Design review of the part built by this model. Coordinates are the model's own, in mm. A direction names the side the tool comes from. Round coordinates to 2 decimals unless told otherwise and drop trailing zeros. Write each loop counter-clockwise with the first axis right and the second up, starting at its lowest first coordinate (ties: lowest second). Pieces come first, ordered by that corner, then holes. Notation, with made-up numbers: (32.25, 3) -> (41.25, 3) arc R24 ccw to (41.25, 18) -> close; hole circle Ø6 at (66, -22). An arc over 180 degrees is marked (long way). One line per question, with ' | ' between items. Start each with the question number.
1) For probe 1 along Y at (x, z) = (3, -3.5); probe 2 along Y at (x, z) = (4, -10); probe 3 along Z at (x, y) = (-0.5, -2.25), list the stretches that pass through material, from the lowest coordinate up.
2) Insertion check: pin 1 Ø2.5 at (y, z) = (5.5, 12) entering from -X; pin 2 Ø4 at (y, z) = (2.5, -4.5) entering from +X; pin 3 Ø2 at (x, z) = (4, -3.5) entering from +Y; pin 4 Ø5 at (x, y) = (5, 6.5) entering from -Z. Each pin has a flat end and moves straight along its axis. Give the tip position at first contact, or say it passes through.
3) Consider section D-D (z = -14.5). Give the boundary of the cut face in (x, y).
4) Mouldability with a two-part tool opening along X and no side actions: class faces 4 (the flat face through (12, 2, 5)), 5 (the flat face through (-15, 6, 0)), 6 (the flat face through (-15, -2, 0)) as +X half, -X half, draft (parallel to the pull), parting line (faces both ways), or undercut.
5) Consider section C-C (y = 2.25). Give the boundary of the cut face in (x, z), then the cut area to 4 significant figures.
6) Consider section B-B (x = -10.5). Give the boundary of the cut face in (y, z), then the cut area to 3 significant figures.
7) Consider section A-A (y = 5.5). Give the boundary of the cut face in (x, z), then the cut area to 3 significant figures.
8) For faces 1 (the flat face through (0, 6, -15)), 2 (the flat face through (0, -1, 2)), 3 (the flat face through (-12, 2, 5)), list the 3-axis set-ups (+Z, -Z, +X, -X, +Y, -Y) from which the entire face can be reached by the end or side of a thin tool; tool diameter is ignored.
```python
from build123d import *

# Parameters (mm, degrees)
SKETCH1_W                = 10
SKETCH1_H                = 15
BOSS_EXTRUDE1_DEPTH      = 4
BOSS_EXTRUDE6_DEPTH      = 8
BOSS_EXTRUDE5_DEPTH      = 15
BOSS_EXTRUDE5_DEPTH_BACK = 15
FILLET2_R                = 1.5
CIRPATTERN2_COUNT        = 4
FILLET2_OF_CIRPATTERN2_R = 1.5
FILLET4_R                = 2


with BuildPart() as part:
    # Sketch1 → Boss-Extrude1 (new body)
    with BuildSketch(Plane(origin=(0, 0, 0), x_dir=(1, 0, 0), z_dir=(0, 1, 0))):
        with Locations((0, 7.5)):
            Rectangle(SKETCH1_W, SKETCH1_H)
        with BuildLine():
            Line((5, 15), (5, 16.248076809))
            ThreePointArc((5, 16.248076809), (0, 17), (-5, 16.248076809))
            Line((-5, 16.248076809), (-5, 15))
            Line((-5, 15), (5, 15))
        make_face()
    boss_extrude1 = extrude(amount=BOSS_EXTRUDE1_DEPTH)

    # Sketch1_6 → Boss-Extrude6 (add)
    with BuildSketch(Plane(origin=(0, 0, 0), x_dir=(1, 0, 0), z_dir=(0, 1, 0))):
        with BuildLine():
            Line((5, 15), (5, 16.248076809))
            ThreePointArc((5, 16.248076809), (0, 17), (-5, 16.248076809))
            Line((-5, 16.248076809), (-5, 15))
            Line((-5, 15), (5, 15))
        make_face()
    boss_extrude6 = extrude(amount=BOSS_EXTRUDE6_DEPTH)

    # Sketch4 → Boss-Extrude5 (add, two sides: drawn at the far end of the back side and taken through both)
    with BuildSketch(Plane.ZY.offset(-BOSS_EXTRUDE5_DEPTH_BACK)):
        Polygon((-2, 0), (-2, -2), (-4.5, -2), (-4.5, -3.436102186), (4.5, -3.436102186), (4.5, -2), (2, -2), (2, 0), align=None)
    extrude(amount=BOSS_EXTRUDE5_DEPTH + BOSS_EXTRUDE5_DEPTH_BACK)

    # Fillet2
    fillet2_edges = [part.edges().sort_by_distance(p)[0] for p in [
        (0, 8, -17),
    ]]
    fillet(fillet2_edges, radius=FILLET2_R)

    # CirPattern2: Boss-Extrude1, Boss-Extrude6 ×4 about axis
    cirpattern2_axis = Axis((0, 0, 0), (0, 1, 0))
    add([boss_extrude1.rotate(cirpattern2_axis, i * 360 / CIRPATTERN2_COUNT) for i in range(1, CIRPATTERN2_COUNT)])
    add([boss_extrude6.rotate(cirpattern2_axis, i * 360 / CIRPATTERN2_COUNT) for i in range(1, CIRPATTERN2_COUNT)])

    # Fillet2 of CirPattern2
    fillet2_of_cirpattern2_edges = [part.edges().sort_by_distance(p)[0] for p in [
        (-17, 8, 0),
        (0, 8, 17),
        (17, 8, 0),
    ]]
    fillet(fillet2_of_cirpattern2_edges, radius=FILLET2_OF_CIRPATTERN2_R)

    # Fillet4
    fillet4_edges = [part.edges().sort_by_distance(p)[0] for p in [
        (-5, 2, -5),
        (5, 2, -5),
        (-5, 2, 5),
        (5, 2, 5),
    ]]
    fillet(fillet4_edges, radius=FILLET4_R)


solid = part.part
```
From the geometry:
1) probe 1: y = -3.44 to -2, 0 to 4 | probe 2: y = 0 to 4 | probe 3: z = -4.5 to 4.5
2) pin 1: passes through | pin 2: stops at x = 16.82 | pin 3: stops at y = 4 | pin 4: stops at z = -16.82
3) outline: (-5, 0) -> (5, 0) -> (5, 4) -> (-5, 4) -> close
4) face 4: draft | face 5: undercut | face 6: -X half
5) outline: (-16.25, -5) -> (-7, -5) arc R2 cw to (-5, -7) -> (-5, -16.25) arc R17 ccw to (5, -16.25) -> (5, -7) arc R2 cw to (7, -5) -> (16.25, -5) arc R17 ccw to (16.25, 5) -> (7, 5) arc R2 cw to (5, 7) -> (5, 16.25) arc R17 ccw to (-5, 16.25) -> (-5, 7) arc R2 cw to (-7, 5) -> (-16.25, 5) arc R17 ccw to start | area: 573.5 mm2
6) outline: (-3.44, -4.5) -> (-2, -4.5) -> (-2, -2) -> (0, -2) -> (0, -5) -> (4, -5) -> (4, 5) -> (0, 5) -> (0, 2) -> (-2, 2) -> (-2, 4.5) -> (-3.44, 4.5) -> close | area: 60.9 mm2
7) outline: (-16.25, -5) -> (-15, -5) -> (-15, 5) -> (-16.25, 5) arc R17 ccw to start; (-5, -16.25) arc R17 ccw to (5, -16.25) -> (5, -15) -> (-5, -15) -> close; (-5, 15) -> (5, 15) -> (5, 16.25) arc R17 ccw to (-5, 16.25) -> close; (15, -5) -> (16.25, -5) arc R17 ccw to (16.25, 5) -> (15, 5) -> close | area: 70.1 mm2
8) face 1: +X, -X, +Y | face 2: +Z, +X, -X | face 3: +Z, -X, +Y, -Y
